Check sheet for the modelled part. Datum: model origin and axes. Units: mm. Coordinates: 2 decimals unless noted, no trailing zeros. Loops run counter-clockwise (first coordinate to the right, second up) from the corner with the lowest first, then second, coordinate; pieces in that order, holes last. Notation, with made-up numbers: M -1.5,70.5 L 30.5,70.5 A17 cw 30.5,75.5 Z; hole C -16,-39 d4. An arc over 180 degrees is marked long. Return JSON: item names as keys, results as strings.
from build123d import *

# Parameters (mm, degrees)
SKETCH1_R           = 1.627
BOSS_EXTRUDE1_DEPTH = 6.35
SKETCH2_W           = 8.278201301
SKETCH2_H           = 8.19304218
CUT_EXTRUDE1_DEPTH  = 3.175


with BuildPart() as part:
    # Sketch1 → Boss-Extrude1 (new body)
    with BuildSketch(Plane.XY):
        with BuildLine():
            Line((-35.456602045, 3.175), (-7.62, 3.175))
            Line((-7.62, 3.175), (-3.175, 3.175))
            ThreePointArc((-3.175, 3.175), (-0.92993597, 2.24506403), (0, 0))
            ThreePointArc((0, 0), (-0.92993597, -2.24506403), (-3.175, -3.175))
            Line((-3.175, -3.175), (-7.62, -3.175))
            Line((-7.62, -3.175), (-35.456602045, -3.175))
            Line((-35.456602045, -3.175), (-61.15130657, -3.175))
            ThreePointArc((-61.15130657, -3.175), (-63.3963706, -2.24506403), (-64.32630657, 0))
            ThreePointArc((-64.32630657, 0), (-63.3963706, 2.24506403), (-61.15130657, 3.175))
            Line((-61.15130657, 3.175), (-35.456602045, 3.175))
        make_face()
        with Locations((-3.175, 0)):
            Circle(SKETCH1_R, mode=Mode.SUBTRACT)
        with Locations((-61.15130657, 0)):
            Circle(SKETCH1_R, mode=Mode.SUBTRACT)
    extrude(amount=BOSS_EXTRUDE1_DEPTH)

    # Sketch2 → Cut-Extrude1 (cut)
    with BuildSketch(Plane.XY.offset(6.35)):
        with Locations((-60.845407221, -0.92152109)):
            Rectangle(SKETCH2_W, SKETCH2_H)
    extrude(amount=-CUT_EXTRUDE1_DEPTH, mode=Mode.SUBTRACT)


solid = part.part
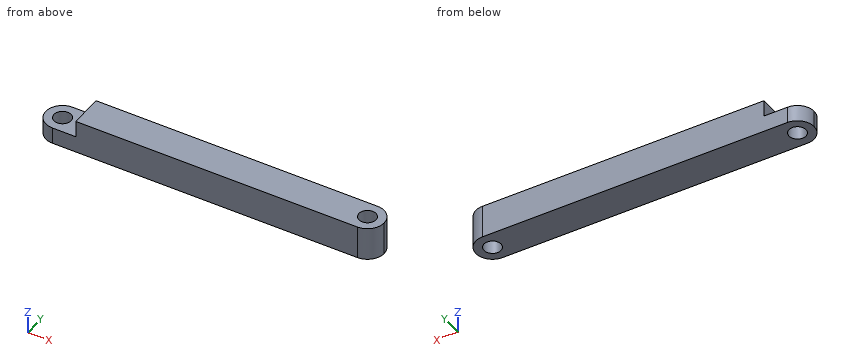
1) Go/stop test with flat-tipped pins: pin 1 Ø1.5 at (x, y) = (-35.5, -2.5) entering from -Z; pin 2 Ø1 at (y, z) = (-1, 4) entering from -X. Record where each tip stops, or that it passes through.
Answers:
{"pin 1": "z = 0", "pin 2": "x = -56.71"}
2) Section check A-A on y = -1. Record the cut outline in (x, z) (3 decimals).
Answers:
{"outline": "M -64.165,0 L -62.435,0 L -62.435,3.175 L -64.165,3.175 Z; M -59.868,0 L -4.458,0 L -4.458,6.35 L -56.706,6.35 L -56.706,3.175 L -59.868,3.175 Z; M -1.892,0 L -0.162,0 L -0.162,6.35 L -1.892,6.35 Z"}
3) Section check C-C on x = -58.5. Record the cut outline in (y, z) (3 decimals), then the cut area to 3 significant figures.
Answers:
{"outline": "M -3.175,0 L 3.175,0 L 3.175,3.175 L -3.175,3.175 Z", "area": "20.2 mm²"}
4) Scan lines: line 1 along X through (y, z) = (-0.5, 3); line 2 along Z through (x, y) = (-58.5, -2.25) (3 decimals); line 3 along Y through (x, z) = (-4.5, 1.75) (3 decimals). Record each from-to range of solid material in increasing order. Write a range as [from, to].
Answers:
{"line 1": "[-64.29, -62.7], [-59.6, -4.72], [-1.63, -0.04]", "line 2": "[0, 3.175]", "line 3": "[-3.175, -0.944], [0.944, 3.175]"}
5) Section check B-B on z = 5. Record the cut outline in (x, y) (3 decimals), then the cut area to 3 significant figures.
Answers:
{"outline": "M -56.706,-3.175 L -3.175,-3.175 A3.175 ccw -3.175,3.175 L -56.706,3.175 Z; hole C -3.175,0 d3.254", "area": "347 mm²"}
